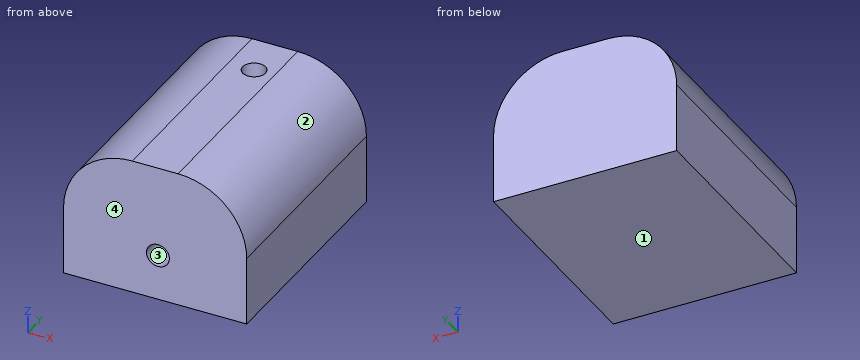
from build123d import *

# Parameters (mm, degrees)
F0_W     = 101.6
F0_H     = 127
F1_DEPTH = 76.2
F2_R     = 38.1
F3_R     = 6.35
F4_DEPTH = 114.3
F5_R     = 6.35
F6_DEPTH = 50.8


with BuildPart() as f1:
    # F0 (on Top) → F1 (new body)
    with BuildSketch(Plane.XY):
        with Locations((-1.54382, 3.250349)):
            Rectangle(F0_W, F0_H)
    extrude(amount=F1_DEPTH)

    # F2
    f2_edges = [f1.edges().sort_by_distance(p)[0] for p in [
        (-52.34382, 3.250349, 76.2),
        (49.25618, 3.250349, 76.2),
    ]]
    fillet(f2_edges, radius=F2_R)

    # F3 (on face) → F4 (cut)
    with BuildSketch(Plane.XZ.offset(60.249651)):
        with Locations((0, 25.4)):
            Circle(F3_R)
    extrude(amount=-F4_DEPTH, mode=Mode.SUBTRACT)

    # F5 (on face) → F6 (cut)
    with BuildSketch(Plane.XY.offset(76.2)):
        with Locations((0, 41.734669)):
            Circle(F5_R)
    extrude(amount=-F6_DEPTH, mode=Mode.SUBTRACT)


solid = f1.part
Geometry check sheet. Reference: the model listing, model coordinates, mm. Face numbers are marked on the shaded views. Round coordinates to 2 decimals unless told otherwise and drop trailing zeros. Loops run counter-clockwise (first coordinate to the right, second up) from the corner with the lowest first, then second, coordinate; pieces in that order, holes last.
Item 1: Cross-section at C-C on z = 48. Record the boundary of the cut face in (x, y).
Item 2: Cross-section at B-B on x = 0. Record the boundary of the cut face in (y, z), then the cut area to 3 significant figures.
Item 3: Thickness scan on line 1 (Z direction, x = 0, y = 7); line 2 (X direction, y = -28, z = 25); line 3 (Y direction, x = 0, z = 43.5). Record the ranges inside material, lowest first.
Item 4: Cross-section at D-D on x = -46. Record the boundary of the cut face in (y, z), then the cut area to 3 significant figures.
Item 5: Cross-section at A-A on y = -15.5. Record the boundary of the cut face in (x, z).
Item 6: Mould release check, pull along Z, two halves, no side actions. Record for the marked faces 1, 2, 3 and 4: pulls with the +Z half, pulls with the -Z half, needs draft (parallel to the pull), parting line crosses it, or undercut.
Answer sheet:
1. outline: (-51.04, -60.25) - (47.95, -60.25) - (47.95, 66.75) - (-51.04, 66.75) - close; hole circle Ø12.7 at (0, 41.73)
2. outline: (-60.25, 0) - (66.75, 0) - (66.75, 76.2) - (48.08, 76.2) - (48.08, 31.75) - (54.05, 31.75) - (54.05, 19.05) - (-60.25, 19.05) - close; (-60.25, 31.75) - (35.38, 31.75) - (35.38, 76.2) - (-60.25, 76.2) - close
2. area: 7,660 mm2
3. line 1: z = 0 to 19.05, 31.75 to 76.2
3. line 2: x = -52.34 to -6.34, 6.34 to 49.26
3. line 3: y = -60.25 to 35.38, 48.08 to 66.75
4. outline: (-60.25, 0) - (66.75, 0) - (66.75, 59.15) - (-60.25, 59.15) - close
4. area: 7,510 mm2
5. outline: (-52.34, 0) - (49.26, 0) - (49.26, 38.1) arc R38.1 ccw to (11.16, 76.2) - (-14.24, 76.2) arc R38.1 ccw to (-52.34, 38.1) - close; hole circle Ø12.7 at (0, 25.4)
6. face 1: pulls with the -Z half
6. face 2: pulls with the +Z half
6. face 3: undercut
6. face 4: needs draft
